```python
from build123d import *

# Parameters (mm, degrees)
SKETCH_1_R      = 2
EXTRUDE_1_DEPTH = 5
SKETCH_2_R      = 5
SKETCH_2_R_2    = 2.5
EXTRUDE_2_DEPTH = 25


with BuildPart() as part:
    # 草图1 → 凸台-拉伸1 (new body)
    with BuildSketch(Plane(origin=(0, 0, 0), x_dir=(1, 0, 0), z_dir=(0, 1, 0))):
        Polygon((0, 6.92820323), (-6, 3.464101615), (-6, -3.464101615), (0, -6.92820323), (6, -3.464101615), (6, 3.464101615), align=None)
        with Locations(Location((0, 0, 0), (0, 0, 270))):
            Circle(SKETCH_1_R, mode=Mode.SUBTRACT)
    extrude(amount=EXTRUDE_1_DEPTH)

    # 草图2 → 凸台-拉伸2 (add)
    with BuildSketch(Plane(origin=(0, 5, 0), x_dir=(1, 0, 0), z_dir=(0, 1, 0))):
        with Locations(Location((0, 0, 0), (0, 0, 270))):
            Circle(SKETCH_2_R)
        with Locations(Location((0, 0, 0), (0, 0, 270))):
            Circle(SKETCH_2_R_2, mode=Mode.SUBTRACT)
    extrude(amount=EXTRUDE_2_DEPTH)


solid = part.part
```
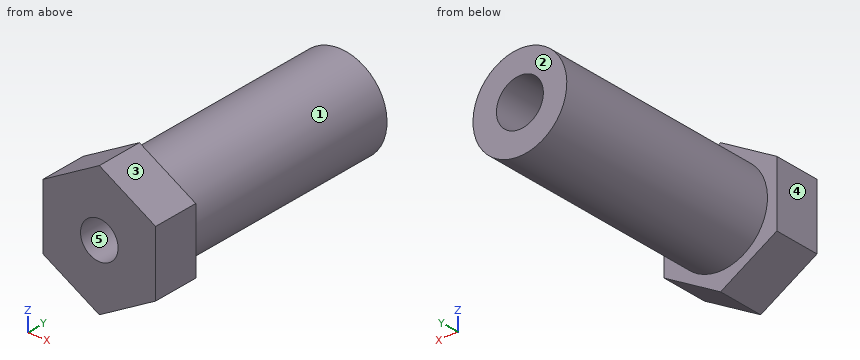
Model file for the job. Use its own axes, mm. Face numbers are marked on the shaded views. A direction names the side the tool comes from. Give positions to 0.01 mm unless a question says otherwise; leave off trailing zeros. Order: outer loops, then holes, each group sorted by start corner. A loop starts at its lowest first (then second) coordinate and runs counter-clockwise, first axis right, second up.
1) Mould opens along Z. For the marked faces 3, 4 and 5 say: +Z half, -Z half, draft (parallel to the pull), parting line (faces both ways), or undercut.
2) Saw through at D-D, the plane z = 4. Write the cut outline in (x, y), then the cut area to 3 significant figures.
3) Saw through at A-A, the plane y = 2.5. Write the cut outline in (x, z), then the cut area to 3 significant figures.
4) Saw through at C-C, the plane x = -1.25. Write the cut outline in (y, z), then the cut area to 3 significant figures.
5) 3-axis set-ups, long thin cutter, end or side, ignore diameter. For the marked faces 1 and 2: which of +Z, -Z, +X, -X, +Y, -Y reach the whole face in a straight line?
6) Saw through at B-B, the plane z = 0. Write the cut outline in (x, y).
7) Pin check, flat tips, straight feed: pin 1 (1.5 mm diameter, centred on y = 10.5, z = -0.5, fed in from +X); pin 2 (5 mm diameter, centred on x = -4.5, y = 27, fed in from -Z); pin 3 (1.5 mm diameter, centred on y = 9.5, z = 4.5, fed in from +X). Stop position of each tip, or through.
8) Wall check: probe 1 along X at (y, z) = (17.5, 0); probe 2 along X at (y, z) = (2.55, 0); probe 3 along Y at (x, z) = (4, 3.5). Give the ranges that are in metal, low to high.
Computed:
1. face 3: +Z half
1. face 4: draft
1. face 5: undercut
2. outline: (-5.07, 0) - (5.07, 0) - (5.07, 5) - (3, 5) - (3, 30) - (-3, 30) - (-3, 5) - (-5.07, 5) - close
2. area: 201 mm2
3. outline: (-6, -3.46) - (0, -6.93) - (6, -3.46) - (6, 3.46) - (0, 6.93) - (-6, 3.46) - close; hole circle Ø4 at (0, 0)
3. area: 112 mm2
4. outline: (0, -6.21) - (5, -6.21) - (5, -4.84) - (30, -4.84) - (30, -2.17) - (5, -2.17) - (5, -1.56) - (0, -1.56) - close; (0, 1.56) - (5, 1.56) - (5, 2.17) - (30, 2.17) - (30, 4.84) - (5, 4.84) - (5, 6.21) - (0, 6.21) - close
4. area: 180 mm2
5. face 1: +Y
5. face 2: +Z, -Z, +X, -X, +Y
6. outline: (-6, 0) - (-2, 0) - (-2, 5) - (-2.5, 5) - (-2.5, 30) - (-5, 30) - (-5, 5) - (-6, 5) - close; (2, 0) - (6, 0) - (6, 5) - (5, 5) - (5, 30) - (2.5, 30) - (2.5, 5) - (2, 5) - close
7. pin 1: stops at x = 5
7. pin 2: stops at z = -4.58
7. pin 3: stops at x = 3.31
8. probe 1: x = -5 to -2.5, 2.5 to 5
8. probe 2: x = -6 to -2, 2 to 6
8. probe 3: y = 0 to 5
